Part model, mm, in its own coordinate system. A direction names the side the tool comes from. Coordinates: 2 decimals unless noted, no trailing zeros. Loops run counter-clockwise (first coordinate to the right, second up) from the corner with the lowest first, then second, coordinate; pieces in that order, holes last. Notation, with made-up numbers: (42, 32.5) - (67, 32.5) arc R18 ccw to (67, 63.5) - close; hole circle Ø9 at (-37.5, -26.5). An arc over 180 degrees is marked (long way). Use a Markdown table: item, result. Add a question column.
1. Band-saw the part on C-C, the plane z = -25. Give the cut face in (x, y).
2. Pull direction Z, two halves, no side cores. Call faces 4 (the cylindrical face through (41.34, 1.52, 30.85)), 5 (the cylindrical face through (-30.18, 1.48, 44.63)), 6 (the flat face through (-75, 1, -38)): pulls with the +Z half, pulls with the -Z half, needs draft (parallel to the pull), parting line crosses it, or undercut.
3. 3-axis set-ups, long thin cutter, end or side, ignore diameter. For faces 1 (the cylindrical face through (65.21, 1.48, 19.92)), 2 (the flat face through (-44, 2, 0)), 3 (the cylindrical face through (30.13, 1.48, -44.61)): which of +Z, -Z, +X, -X, +Y, -Y reach the whole face in a straight line?
4. Band-saw the part on D-D, the plane y = 0.95. Count the separate pieces of the cut face and the enclosed holes in it, plus the area to 3 significant figures.
5. Band-saw the part on A-A, the plane z = 7.5. Give the cut face in (x, y).
6. Wall check: probe 1 along X at (y, z) = (1.45, -15); probe 2 along X at (y, z) = (1.5, 20); probe 3 along X at (y, z) = (0.85, 40). Give the ranges that are in metal, low to high. Write a range as [from, to].
7. Band-saw the part on B-B, the plane x = -20. Give the cut face in (y, z), plus the area to 3 significant figures.
from build123d import *

# Parameters (mm, degrees)
CROQUIS1_W              = 150
CROQUIS1_H              = 90
CROQUIS1_R              = 1.5875
SALIENTE_EXTRUIR1_DEPTH = 3
CROQUIS2_R              = 1.5875
CORTAR_EXTRUIR1_DEPTH   = 3
CROQUIS3_R              = 1.6
ANCLAJE_BANDA_DEPTH     = 10
CROQUIS4_R              = 1.6
ESPACIO_CENTRO_DEPTH    = 10
CROQUIS5_R              = 1.6
ESPACIO_EXTERNO_DEPTH   = 10
CROQUIS6_W              = 12
CROQUIS6_H              = 45
QUITA_PESO_DEPTH        = 10
REDONDEO1_R             = 5


with BuildPart() as part:
    # Croquis1 → Saliente-Extruir1 (new body)
    with BuildSketch(Plane(origin=(0, 0, 0), x_dir=(1, 0, 0), z_dir=(0, 1, 0))):
        Rectangle(CROQUIS1_W, CROQUIS1_H)
        with Locations(Location((-60, 30, 0), (0, 0, 270))):
            Circle(CROQUIS1_R, mode=Mode.SUBTRACT)
        with Locations(Location((-60, -30, 0), (0, 0, 270))):
            Circle(CROQUIS1_R, mode=Mode.SUBTRACT)
        with Locations(Location((60, -30, 0), (0, 0, 270))):
            Circle(CROQUIS1_R, mode=Mode.SUBTRACT)
        with Locations(Location((60, 30, 0), (0, 0, 270))):
            Circle(CROQUIS1_R, mode=Mode.SUBTRACT)
    extrude(amount=SALIENTE_EXTRUIR1_DEPTH)

    # Croquis2 → Cortar-Extruir1 (cut)
    with BuildSketch(Plane(origin=(0, 3, 0), x_dir=(1, 0, 0), z_dir=(0, 1, 0))):
        with Locations(Location((-40, 30, 0), (0, 0, 270))):
            Circle(CROQUIS2_R)
        with Locations(Location((-40, -30, 0), (0, 0, 270))):
            Circle(CROQUIS2_R)
        with Locations(Location((40, -30, 0), (0, 0, 270))):
            Circle(CROQUIS2_R)
        with Locations(Location((40, 30, 0), (0, 0, 270))):
            Circle(CROQUIS2_R)
    extrude(amount=-CORTAR_EXTRUIR1_DEPTH, mode=Mode.SUBTRACT)

    # Croquis3 → Anclaje_Banda (cut)
    with BuildSketch(Plane(origin=(0, 3, 0), x_dir=(1, 0, 0), z_dir=(0, 1, 0))):
        with Locations(Location((6, -25, 0), (0, 0, 270))):
            Circle(CROQUIS3_R)
        with Locations(Location((6, 25, 0), (0, 0, 270))):
            Circle(CROQUIS3_R)
    extrude(amount=-ANCLAJE_BANDA_DEPTH, mode=Mode.SUBTRACT)

    # Croquis4 → Espacio_Centro (cut)
    with BuildSketch(Plane(origin=(0, 3, 0), x_dir=(1, 0, 0), z_dir=(0, 1, 0))):
        with Locations(Location((20, -20, 0), (0, 0, 270))):
            Circle(CROQUIS4_R)
        with Locations(Location((-20, -20, 0), (0, 0, 270))):
            Circle(CROQUIS4_R)
        with Locations(Location((-20, 20, 0), (0, 0, 270))):
            Circle(CROQUIS4_R)
        with Locations(Location((20, 20, 0), (0, 0, 270))):
            Circle(CROQUIS4_R)
    extrude(amount=-ESPACIO_CENTRO_DEPTH, mode=Mode.SUBTRACT)

    # Croquis5 → Espacio_externo (cut)
    with BuildSketch(Plane(origin=(0, 3, 0), x_dir=(1, 0, 0), z_dir=(0, 1, 0))):
        with Locations(Location((-70, 40, 0), (0, 0, 270))):
            Circle(CROQUIS5_R)
        with Locations(Location((70, 40, 0), (0, 0, 270))):
            Circle(CROQUIS5_R)
        with Locations(Location((70, -40, 0), (0, 0, 270))):
            Circle(CROQUIS5_R)
        with Locations(Location((-70, -40, 0), (0, 0, 270))):
            Circle(CROQUIS5_R)
    extrude(amount=-ESPACIO_EXTERNO_DEPTH, mode=Mode.SUBTRACT)

    # Croquis6 → Quita_peso (cut)
    with BuildSketch(Plane(origin=(0, 3, 0), x_dir=(1, 0, 0), z_dir=(0, 1, 0))):
        Polygon((-75, 35), (-65, 20), (-65, -20), (-75, -35), align=None)
        Polygon((75, 35), (75, -35), (65, -20), (65, 20), align=None)
        with Locations((-50, 0)):
            Rectangle(CROQUIS6_W, CROQUIS6_H)
        with Locations((50, 0)):
            Rectangle(CROQUIS6_W, CROQUIS6_H)
        Polygon((-30, 45), (-20, 35), (20, 35), (30, 45), align=None)
        Polygon((20, -35), (30, -45), (-30, -45), (-20, -35), align=None)
    extrude(amount=-QUITA_PESO_DEPTH, mode=Mode.SUBTRACT)

    # Redondeo1
    redondeo1_edges = [part.edges().sort_by_distance(p)[0] for p in [
        (-75, 1.5, 35),
        (-75, 1.5, -35),
        (-65, 1.5, -20),
        (-65, 1.5, 20),
        (-30, 1.5, 45),
        (30, 1.5, 45),
        (-30, 1.5, -45),
        (30, 1.5, -45),
        (75, 1.5, 35),
        (75, 1.5, -35),
        (-20, 1.5, 35),
        (20, 1.5, 35),
        (20, 1.5, -35),
        (-20, 1.5, -35),
        (56, 1.5, -22.5),
        (56, 1.5, 22.5),
        (44, 1.5, 22.5),
        (44, 1.5, -22.5),
        (-44, 1.5, -22.5),
        (-44, 1.5, 22.5),
        (-56, 1.5, 22.5),
        (-56, 1.5, -22.5),
        (65, 1.5, 20),
        (65, 1.5, -20),
        (75, 1.5, 45),
        (-75, 1.5, 45),
        (-75, 1.5, -45),
        (75, 1.5, -45),
    ]]
    fillet(redondeo1_edges, radius=REDONDEO1_R)


solid = part.part
Geometry check:
| question | item | result |
|---|---|---|
| 1 | outline | (-68.33, 0) - (4.4, 0) - (4.4, 3) - (-68.33, 3) - close; (7.6, 0) - (68.33, 0) - (68.33, 3) - (7.6, 3) - close |
| 2 | face 4 | undercut |
| 2 | face 5 | pulls with the +Z half |
| 2 | face 6 | needs draft |
| 3 | face 1 | +X, +Y, -Y |
| 3 | face 2 | +Y, -Y |
| 3 | face 3 | -Z, +Y, -Y |
| 4 | separate pieces | 1 |
| 4 | enclosed holes | 20 |
| 4 | area | 10,200 mm^2 |
| 5 | outline | (-65, 0) - (-56, 0) - (-56, 3) - (-65, 3) - close; (-44, 0) - (44, 0) - (44, 3) - (-44, 3) - close; (56, 0) - (65, 0) - (65, 3) - (56, 3) - close |
| 6 | probe 1 | x = [-65, -56], [-44, 44], [56, 65] |
| 6 | probe 2 | x = [-65.23, -55.33], [-44.67, -21.6], [-18.4, 18.4], [21.6, 44.67], [55.33, 65.23] |
| 6 | probe 3 | x = [-75, -71.6], [-68.4, -25], [25, 68.4], [71.6, 75] |
| 7 | outline | (0, -35.45) - (3, -35.45) - (3, -21.6) - (0, -21.6) - close; (0, -18.4) - (3, -18.4) - (3, 18.4) - (0, 18.4) - close; (0, 21.6) - (3, 21.6) - (3, 35.45) - (0, 35.45) - close |
| 7 | area | 193 mm^2 |
